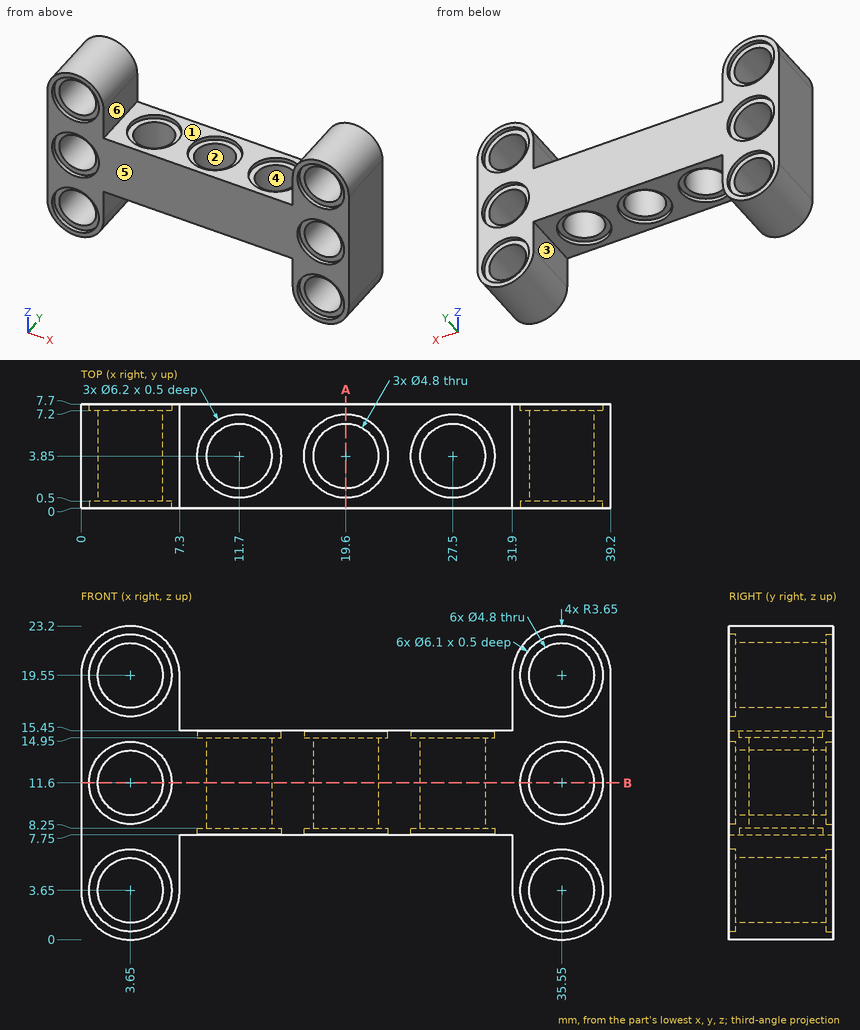
Job drawing, mm, ordinate dimensions from the low corner. One solid piece. A direction names the side the tool comes from. Round coordinates to 2 decimals unless told otherwise and drop trailing zeros. Loops run counter-clockwise (first coordinate to the right, second up) from the corner with the lowest first, then second, coordinate; pieces in that order, holes last. Notation, with made-up numbers: (27.5, -36.75) -> (75.5, -36.75) arc R25 ccw to (75.5, -7.75) -> close; hole circle Ø6 at (22, -19). An arc over 180 degrees is marked (long way). Use a Markdown table: item, result.
1) Cut at B-B, the plane z = 11.6. State how many separate pieces and enclosed holes the cut face has, and give its area (3 significant figures).
The answers:
| item | result |
|---|---|
| separate pieces | 3 |
| enclosed holes | 3 |
| area | 171 mm2 |
2) Cut at A-A, the plane x = 19.6. List the corners of the cut face in (y, z).
The answers:
| item | result |
|---|---|
| outline | (0, 7.75) -> (0.75, 7.75) -> (0.75, 8.25) -> (1.45, 8.25) -> (1.45, 14.95) -> (0.75, 14.95) -> (0.75, 15.45) -> (0, 15.45) -> close; (6.25, 8.25) -> (6.95, 8.25) -> (6.95, 7.75) -> (7.7, 7.75) -> (7.7, 15.45) -> (6.95, 15.45) -> (6.95, 14.95) -> (6.25, 14.95) -> close |
3) Tool access for the marked faces 1, 2 and 3: list every direction of +Z, -Z, +X, -X, +Y, -Y with a clear straight run to the whole face (end or side of a thin tool).
The answers:
| item | result |
|---|---|
| face 1 | +Z, +Y, -Y |
| face 2 | +Z, -Z |
| face 3 | -Z, +Y, -Y |
4) Pull direction Y, two halves, no side cores. Call the marked faces 4, 5 and 6: pulls with the +Y half, pulls with the -Y half, needs draft (parallel to the pull), parting line crosses it, or undercut.
The answers:
| item | result |
|---|---|
| face 4 | undercut |
| face 5 | pulls with the -Y half |
| face 6 | needs draft |
5) Probe line 1 (X direction, y = 4.25, z = 19.55); line 2 (Z direction, x = 35.55, y = 0.1); line 3 (X direction, y = 6.75, z = 11.75). List the from-to ranges inside material, lowest first. Write a range as [from, to].
The answers:
| item | result |
|---|---|
| line 1 | x = [0, 1.25], [6.05, 7.3], [31.9, 33.15], [37.95, 39.2] |
| line 2 | z = [0, 0.6], [6.7, 8.55], [14.65, 16.5], [22.6, 23.2] |
| line 3 | x = [0, 1.25], [6.05, 33.15], [37.95, 39.2] |
6) Drop flat-ended pins along their axis: pin 1 Ø2 at (x, y) = (33, 3.5) entering from -Z; pin 2 Ø1 at (x, y) = (12.5, 1.5) entering from -Z; pin 3 Ø6 at (x, z) = (35.55, 3.65) entering from -Y; pin 4 Ø6.5 at (x, z) = (4.5, 19) entering from -Y. Give the stop position or say it passes through.
The answers:
| item | result |
|---|---|
| pin 1 | stops at z = 0.35 |
| pin 2 | stops at z = 8.25 |
| pin 3 | stops at y = 0.5 |
| pin 4 | stops at y = 0 |
